The figure shows three views and two pictorial views of one solid part (mm, origin at its lowest corner). Answer the questions. Coordinates: 2 decimals unless noted, no trailing zeros. Order: outer loops, then holes, each group sorted by start corner. A loop starts at its lowest first (then second) coordinate and runs counter-clockwise, first axis right, second up. Notation, with made-up numbers: (0.25, -10.5) - (12.25, -10.5) arc R15 cw to (12.25, 9.5) - close; hole circle Ø1 at (-36.75, 47.5). An arc over 180 degrees is marked (long way). Use one line per item in the form item = value. Start each with the question number.
Item 1: Each of these flat-tipped pins is pushed along its axis until it touches: pin 1 Ø1 at (x, y) = (5, 178.5) entering from +Z; pin 2 Ø1.5 at (x, z) = (10, 6) entering from -Y; pin 3 Ø1 at (y, z) = (71, 4.5) entering from -X. Where does it stop, or does it pass through?
Item 2: Consider line 1 along X through (y, z) = (310, 7); line 2 along X through (y, z) = (42.5, 6.75). Determine where each line is inside the solid, lowest interval first. Write a range as [from, to].
Item 3: Section A-A, the plane y = 369 is taken. Write down the section's boundary in (x, z).
Item 4: Section B-B, the plane z = 2.75 is taken. Write down the section's boundary in (x, y).
Item 5: Section C-C, the plane x = 4.5 is taken. Write down the section's boundary in (y, z).
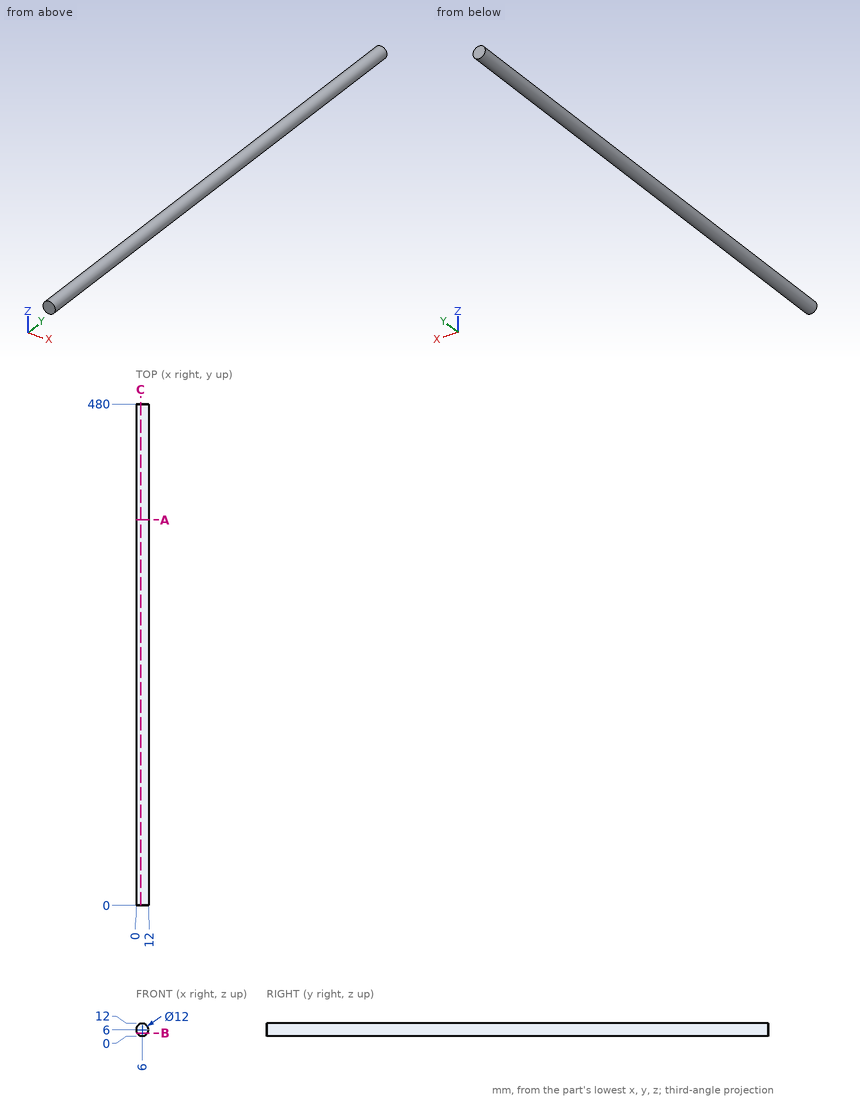
Response:
q1.pin_1 = 11.98
q1.pin_2 = 0
q1.pin_3 = 0.08
q2.line_1 = [0.08, 11.92]
q2.line_2 = [0.05, 11.95]
q3.outline = circle Ø12 at (6, 6)
q4.outline = (0.96, 0) - (11.04, 0) - (11.04, 480) - (0.96, 480) - close
q5.outline = (0, 0.19) - (480, 0.19) - (480, 11.81) - (0, 11.81) - close
